```python
from build123d import *

# Parameters (mm, degrees)
SKETCH_1_W     = 613
SKETCH_1_H     = 7.5
FILLET_1_R     = 0.3
CHAMFER_1_SIZE = 0.5


with BuildPart() as part:
    # 스케치1 → 회전1 (revolve)
    with BuildSketch(Plane.XY, mode=Mode.PRIVATE) as revolve_1_sk:
        with Locations((306.5, 3.75)):
            Rectangle(SKETCH_1_W, SKETCH_1_H)
    revolve(revolve_1_sk.sketch.rotate(Axis((0, 0, 0), (1, 0, 0)), 90), axis=Axis((0, 0, 0), (1, 0, 0)))

    # 스케치2 → 회전3 (revolve)
    with BuildSketch(Plane.XY, mode=Mode.PRIVATE) as revolve_3_sk:
        Polygon((613, 5), (618, 5), (618, 6), (623, 6), (623, 7.5), (628, 7.5), (628, 6.2), (628.2, 6), (657.5, 6), (658, 5.5), (658, 5), (673, 5), (673, 0), (613, 0), align=None)
    revolve(revolve_3_sk.sketch.rotate(Axis((613, 0, 0), (1, 0, 0)), 90), axis=Axis((613, 0, 0), (1, 0, 0)))

    # 스케치3 → 회전4 (revolve)
    with BuildSketch(Plane.XY, mode=Mode.PRIVATE) as revolve_4_sk:
        Polygon((0, 5), (-8, 5), (-8, 4.8), (-9.15, 4.8), (-9.15, 5), (-12, 5), (-12, 0), (0, 0), align=None)
    revolve(revolve_4_sk.sketch.rotate(Axis((0, 0, 0), (-1, 0, 0)), 90), axis=Axis((0, 0, 0), (-1, 0, 0)))

    # 필렛1
    fillet_1_edges = [part.edges().sort_by_distance(p)[0] for p in [
        (0, 0, 5),
    ]]
    fillet(fillet_1_edges, radius=FILLET_1_R)

    # 모따기1
    chamfer_1_edges = [part.edges().sort_by_distance(p)[0] for p in [
        (-12, 0, 5),
        (0, 0, -7.5),
    ]]
    chamfer(chamfer_1_edges, length=CHAMFER_1_SIZE)


solid = part.part
```
Build history of the part. All positions in model axes, mm. A direction names the side the tool comes from. Give positions to 0.01 mm unless a question says otherwise; leave off trailing zeros. Order: outer loops, then holes, each group sorted by start corner. A loop starts at its lowest first (then second) coordinate and runs counter-clockwise, first axis right, second up. Notation, with made-up numbers: M -8,-19.5 L 1,-19.5 A12 ccw 1,2.5 Z; hole C 35.25,-30.5 d2. An arc over 180 degrees is marked long. Return JSON: item names as keys, results as strings.
Q1. 3-axis set-ups, long thin cutter, end or side, ignore diameter. For faces 5 (the face through (613, 5, -2)), 6 (the face through (628, -6, -3)), 7 (the face through (311.038, -6.324, 4.032)): which of +Z, -Z, +X, -X, +Y, -Y reach the whole face in a straight line?
Answer list:
{"face 5": "none", "face 6": "+X", "face 7": "+X, -X"}
Q2. Two-plate mould, pull along X, no slides. Class faces 1 (the face through (618, -4, 4)), 2 (the face through (625.535, -6.324, 4.032)), 3 (the face through (623, -6, -2)), 4 (the face through (0, -5, -3)): pulls with the +X half, pulls with the -X half, needs draft (parallel to the pull), parting line crosses it, or undercut.
Answer list:
{"face 1": "undercut", "face 2": "needs draft", "face 3": "undercut", "face 4": "pulls with the -X half"}
Q3. Flat gauge pins, fed straight in: pin 1 (2 mm diameter, centred on y = -4.5, z = -4.5, fed in from -X); pin 2 (1.5 mm diameter, centred on x = 60, z = -1, fed in from -Y); pin 3 (1 mm diameter, centred on x = 302.5, y = -2, fed in from +Z). Where does each tip first touch, or does it go through?
Answer list:
{"pin 1": "stops at x = 0", "pin 2": "stops at y = -7.5", "pin 3": "stops at z = 7.35"}
Q4. Wall check: probe 1 along X at (y, z) = (1.75, 6.75); probe 2 along X at (y, z) = (-5, -2.5); probe 3 along Z at (x, y) = (225, 2.75). Give the ranges that are in metal, low to high. Write a range as from..to.
Answer list:
{"probe 1": "x = 0..613, 623..628", "probe 2": "x = 0..613, 618..657.91", "probe 3": "z = -6.98..6.98"}
Q5. Band-saw the part on A-A (x = 178). Give the cut face in (y, z), then the cut area to 3 significant figures.
Answer list:
{"outline": "C 0,0 d15", "area": "177 mm^2"}
